Autodesk Fusion 360 part; units mm, degrees
sketch "Esboço1" plane through (0, 0, 0) normal (0, 0, 1) x (1, 0, 0)
  line L0 (0, 0) -> (39, 0)
  line L1 (39, 0) -> (39, 70)
  line L2 (0, 0) -> (0, 70)
  line L3 (0, 70) -> (39, 70)
  dimension "d1" = 39
  dimension "d2" = 70
extrude "Extrusão1" add sketch "Esboço1" along normal blind 10
sketch "Esboço3" plane through (0, 0, 0) normal (0, 0, -1) x (1, 0, 0)
  line L0 (39, 0) -> (0, 0)
  line L1 (0, 0) -> (0, -70)
  line L2 (0, -70) -> (39, -70)
  line L3 (39, -70) -> (39, 0)
  line L4 (39, 0) -> (39, -35) construction
  line L5 (39, -35) -> (0, -35) construction
  circle A0 centre (19.5, -35) radius 3.5
  dimension "d5" = 7
extrude "Extrusão2" cut sketch "Esboço3" against normal blind 10 contours A0
sketch "Esboço4" plane through (0, 0, 0) normal (0, 0, -1) x (1, 0, 0)
  circle A0 centre (19.5, -35) radius 3.5
  line L0 (39, 0) -> (0, 0)
  line L1 (0, 0) -> (0, -70)
  line L2 (0, -70) -> (39, -70)
  line L3 (39, -70) -> (39, 0)
  circle A1 centre (19.5, -35) radius 6.5
  dimension "d8" = 13
extrude "Extrusão3" cut sketch "Esboço4" against normal blind 3.3 contours A1
fillet "Arredondamento1" radius 5 2 edges at (19.5, 70, 10) (19.5, 70, 0)
sketch "Esboço5" plane through (0, 0, 0) normal (-1, 0, 0) x (0, -1, 0)
  arc A0 (-65, 10) -> (-65, 0) centre (-65, 5) ccw
  line L0 (-65, 0) -> (0, 0)
  line L1 (0, 0) -> (0, 10)
  line L2 (0, 10) -> (-65, 10)
  circle A1 centre (-65, 5) radius 2
  dimension "d13" = 4
extrude "Extrusão4" cut sketch "Esboço5" against normal blind 40 contours A1
fillet "Arredondamento2" radius 5 2 edges at (19.5, 0, 10) (19.5, 0, 0)
sketch "Esboço6" plane through (0, 0, 0) normal (-1, 0, 0) x (0, -1, 0)
  circle A0 centre (-65, 5) radius 2
  arc A1 (-5, 0) -> (-5, 10) centre (-5, 5) ccw
  line L0 (-5, 10) -> (-65, 10)
  arc A2 (-65, 10) -> (-65, 0) centre (-65, 5) ccw
  line L1 (-65, 0) -> (-5, 0)
  circle A3 centre (-5, 5) radius 2
  dimension "d18" = 4
extrude "Extrusão5" cut sketch "Esboço6" against normal blind 40 contours A3
fillet "Arredondamento3" radius 0.5 3 edges at (13.4399, 32.6495, 0) (16.2369, 36.2657, 3.3) (16.2369, 36.2657, 10)
fillet "Arredondamento4" radius 1 8 edges at (39, 70, 5) (39, 35, 10) (39, 0, 5) (39, 35, 0) (0, 35, 10) (0, 0, 5) (0, 35, 0) (0, 70, 5)
CAD build for the part. Positions are in the model's coordinates, mm. A direction names the side the tool comes from. Round coordinates to 2 decimals unless told otherwise and drop trailing zeros. Order: outer loops, then holes, each group sorted by start corner. A loop starts at its lowest first (then second) coordinate and runs counter-clockwise, first axis right, second up. Notation, with made-up numbers: M -22,-5.5 L 18,-5.5 A27 cw 18,10.5 Z; hole C -19,-33 d8. An arc over 180 degrees is marked long. Use one line per item in the form item = value.
Q1. Which spindle directions (+Z, -Z, +X, -X, +Y, -Y) get a long thin tool onto all of the face, cutting with end or side? Do faces 1 (the cylindrical face through (14.709, 30.607, 1.88)), 2 (the cylindrical face through (20, 2, 9)). Say none if no direction does.
Recorded:
face_1 = -Z
face_2 = +Z, +X, -X, -Y
Q2. Saw through at A-A on x = 19.5. State how many separate pieces and enclosed holes the cut face has, then the cut area to 3 significant figures.
Recorded:
separate_pieces = 2
enclosed_holes = 2
area = 563 mm^2
Q3. Probe L1, parallel to Z at x = 14.5, y = 5; L2, parallel to Y at x = 28, z = 6.75; L3, parallel to Y at x = 21.5, z = 3.5. List the from-to ranges inside material, lowest first.
Recorded:
L1 = 0 to 3, 7 to 10
L2 = 0.32 to 4.03, 5.97 to 64.03, 65.97 to 69.68
L3 = 0.23 to 3.68, 6.32 to 32.01, 37.99 to 63.68, 66.32 to 69.77
Q4. Saw through at B-B on y = 35. Give the cut face in (x, z), then the cut area to 3 significant figures.
Recorded:
outline = M 0,1 A1 ccw 1,0 L 12.5,0 A0.5 ccw 13,0.5 L 13,3.3 L 15.5,3.3 A0.5 ccw 16,3.8 L 16,9.5 A0.5 ccw 15.5,10 L 1,10 A1 ccw 0,9 Z; M 23,3.8 A0.5 ccw 23.5,3.3 L 26,3.3 L 26,0.5 A0.5 ccw 26.5,0 L 38,0 A1 ccw 39,1 L 39,9 A1 ccw 38,10 L 23.5,10 A0.5 ccw 23,9.5 Z
area = 299 mm^2
Q5. Two-plate mould, pull along Y, no slides. Class faces 3 (the cylindrical face through (20, 1, 2)), 4 (the flat face through (39, 35, 5)), 5 (the flat face through (24, 35, 3.3)): +Y half, -Y half, draft (parallel to the pull), parting line (faces both ways), or undercut.
Recorded:
face_3 = -Y half
face_4 = draft
face_5 = undercut
Q6. Flat gauge pins, fed straight in: P1, Ø2, axis at x = 27.5, z = 1.5, coming from the -Y side; P2, Ø3, axis at y = 5, z = 5, coming from the +X side; P3, Ø6.5, axis at x = 21, y = 36, coming from the -Z side; P4, Ø3, axis at x = 6.5, z = 2.5, coming from the +Y side. Where does each tip first touch, or does it go through?
Recorded:
P1 = 0.67
P2 = through
P3 = 3.3
P4 = 69.9
